Autodesk Inventor part; units mm, degrees
ref_plane "YZ Plane" through (0, 0, 0) normal (1, 0, 0) x (0, 1, 0)
ref_plane "XZ Plane" through (0, 0, 0) normal (0, 1, 0) x (-1, 0, 0)
ref_plane "XY Plane" through (0, 0, 0) normal (0, 0, 1) x (1, 0, 0)
sketch "Эскиз1" plane through (0, 0, 0) normal (1, 0, 0) x (0, 1, 0)
  line L0 (97.2644, 106.089) -> (-2.7356, 106.089)
  line L1 (-2.7356, 106.089) -> (-2.7356, -97.911)
  line L2 (-2.7356, -97.911) -> (97.2644, -97.911)
  line L3 (97.2644, -97.911) -> (97.2644, 106.089)
  line L4 (-2.7356, 106.089) -> (3.2644, 106.089)
  line L5 (3.2644, 106.089) -> (3.2644, 66.089)
  line L6 (3.2644, 66.089) -> (-2.7356, 66.089)
  line L7 (-2.7356, 66.089) -> (-2.7356, 106.089)
  line L8 (3.2644, 66.089) -> (-2.7356, 66.089)
  line L9 (-2.7356, 66.089) -> (-2.7356, 36.089)
  line L10 (-2.7356, 36.089) -> (3.2644, 36.089)
  line L11 (3.2644, 36.089) -> (3.2644, 66.089)
  line L12 (-2.7356, 36.089) -> (3.2644, 36.089)
  line L13 (3.2644, 36.089) -> (3.2644, -27.911)
  line L14 (3.2644, -27.911) -> (-2.7356, -27.911)
  line L15 (-2.7356, -27.911) -> (-2.7356, 36.089)
  line L16 (3.2644, -27.911) -> (-2.7356, -27.911)
  line L17 (-2.7356, -27.911) -> (-2.7356, -57.911)
  line L18 (-2.7356, -57.911) -> (3.2644, -57.911)
  line L19 (3.2644, -57.911) -> (3.2644, -27.911)
  line L20 (3.2644, -57.911) -> (-2.7356, -57.911)
  line L21 (-2.7356, -57.911) -> (-2.7356, -97.911)
  line L22 (-2.7356, -97.911) -> (3.2644, -97.911)
  line L23 (3.2644, -97.911) -> (3.2644, -57.911)
  line L24 (3.2644, 91.089) -> (-2.7356, 91.089)
  line L25 (-2.7356, 91.089) -> (-2.7356, 81.089)
  line L26 (-2.7356, 81.089) -> (3.2644, 81.089)
  line L27 (3.2644, 81.089) -> (3.2644, 91.089)
  line L28 (3.2644, -72.911) -> (-2.7356, -72.911)
  line L29 (-2.7356, -72.911) -> (-2.7356, -82.911)
  line L30 (-2.7356, -82.911) -> (3.2644, -82.911)
  line L31 (3.2644, -82.911) -> (3.2644, -72.911)
  point P0 (0, 0)
  point P1 (-2.7356, 66.089)
  point P2 (3.2644, 36.089)
  point P3 (-2.7356, -27.911)
  point P4 (0.2644, 91.089)
  point P5 (0.2644, 81.089)
  point P6 (0.2644, 66.089)
  point P7 (0.2644, -57.911)
  point P8 (0.2644, -72.911)
  point P9 (0.2644, -82.911)
  dimension "d0" = 204
  dimension "d1" = 100
  dimension "d2" = 40
  dimension "d3" = 30
  dimension "d4" = 30
  dimension "d5" = 40
  dimension "d8" = 6
  dimension "d41" = 10
  dimension "d42" = 15
  dimension "d43" = 15
  dimension "d44" = 10
extrude "Выдавливание1" add sketch "Эскиз1" along normal blind 6 contours L3 L2 L23 L19 L13 L11 L5 L0 | L5 L26 L1 L24 | L30 L1 L28 L23 | L11 L10 L1 L6 | L18 L1 L14 L19
sketch "Эскиз2" plane through (6, 0, 0) normal (1, 0, 0) x (0, 0, -1)
  line L0 (-106.089, 97.2644) -> (-106.089, 3.2644)
  line L1 (-106.089, 3.2644) -> (-100.089, 3.2644)
  line L2 (-100.089, 3.2644) -> (-100.089, 13.2644)
  line L3 (-100.089, 13.2644) -> (-106.089, 13.2644)
  line L4 (-106.089, 13.2644) -> (-106.089, 3.2644)
  line L5 (-106.089, 33.2644) -> (-100.089, 33.2644)
  line L6 (-100.089, 33.2644) -> (-100.089, 13.2644)
  line L7 (-100.089, 13.2644) -> (-106.089, 13.2644)
  line L8 (-106.089, 13.2644) -> (-106.089, 33.2644)
  line L9 (-100.089, 33.2644) -> (-106.089, 33.2644)
  line L10 (-106.089, 33.2644) -> (-106.089, 67.2644)
  line L11 (-106.089, 67.2644) -> (-100.089, 67.2644)
  line L12 (-100.089, 67.2644) -> (-100.089, 33.2644)
  line L13 (-100.089, 67.2644) -> (-106.089, 67.2644)
  line L14 (-106.089, 67.2644) -> (-106.089, 87.2644)
  line L15 (-106.089, 87.2644) -> (-100.089, 87.2644)
  line L16 (-100.089, 87.2644) -> (-100.089, 67.2644)
  line L17 (-100.089, 87.2644) -> (-106.089, 87.2644)
  line L18 (-106.089, 87.2644) -> (-106.089, 97.2644)
  line L19 (-106.089, 97.2644) -> (-100.089, 97.2644)
  line L20 (-100.089, 97.2644) -> (-100.089, 87.2644)
  line L21 (57.911, 3.2644) -> (97.911, 3.2644)
  line L22 (97.911, 3.2644) -> (91.911, 3.2644)
  line L23 (91.911, 3.2644) -> (91.911, 13.2644)
  line L24 (91.911, 13.2644) -> (97.911, 13.2644)
  line L25 (97.911, 13.2644) -> (97.911, 3.2644)
  line L26 (97.911, 13.2644) -> (91.911, 13.2644)
  line L27 (91.911, 13.2644) -> (91.911, 33.2644)
  line L28 (91.911, 33.2644) -> (97.911, 33.2644)
  line L29 (97.911, 33.2644) -> (97.911, 13.2644)
  line L30 (97.911, 33.2644) -> (91.911, 33.2644)
  line L31 (91.911, 33.2644) -> (91.911, 67.2644)
  line L32 (91.911, 67.2644) -> (97.911, 67.2644)
  line L33 (97.911, 67.2644) -> (97.911, 33.2644)
  line L34 (97.911, 67.2644) -> (91.911, 67.2644)
  line L35 (91.911, 67.2644) -> (91.911, 87.2644)
  line L36 (91.911, 87.2644) -> (97.911, 87.2644)
  line L37 (97.911, 87.2644) -> (97.911, 67.2644)
  line L38 (97.911, 87.2644) -> (91.911, 87.2644)
  line L39 (91.911, 87.2644) -> (91.911, 97.2644)
  line L40 (91.911, 97.2644) -> (97.911, 97.2644)
  line L41 (97.911, 97.2644) -> (97.911, 87.2644)
  point P0 (0, 0)
  point P1 (91.911, 3.2644)
  dimension "d9" = 10
  dimension "d10" = 20
  dimension "d11" = 10
  dimension "d12" = 20
  dimension "d13" = 34
  dimension "d14" = 6
  dimension "d15" = 10
  dimension "d16" = 20
  dimension "d17" = 20
  dimension "d18" = 10
  dimension "d19" = 34
  dimension "d20" = 6
extrude "Выдавливание2" cut sketch "Эскиз2" against normal through all contours L19 L20 L15 L0 | L11 L12 L5 L0 | L3 L2 L1 L0 | L23 L24 L25 L21 | L31 L32 L33 L28 | L39 L40 L41 L36
sketch "Эскиз4" plane through (6, 0, 0) normal (1, 0, 0) x (0, 0, -1)
  line L0 (-36.089, 3.2644) -> (27.911, 3.2644)
  line L1 (-19, 3.2644) -> (-16, 3.2644)
  line L2 (-16, 3.2644) -> (-16, 13.2644)
  line L3 (-16, 13.2644) -> (-19, 13.2644)
  line L4 (-19, 13.2644) -> (-19, 3.2644)
  line L5 (-21, 7.6644) -> (-14, 7.6644)
  line L6 (-14, 7.6644) -> (-14, 5.2644)
  line L7 (-14, 5.2644) -> (-21, 5.2644)
  line L8 (-21, 5.2644) -> (-21, 7.6644)
  line L9 (7, 3.2644) -> (4, 3.2644)
  line L10 (4, 3.2644) -> (4, 13.2644)
  line L11 (4, 13.2644) -> (7, 13.2644)
  line L12 (7, 13.2644) -> (7, 3.2644)
  line L13 (2, 7.6644) -> (9, 7.6644)
  line L14 (9, 7.6644) -> (9, 5.2644)
  line L15 (9, 5.2644) -> (2, 5.2644)
  line L16 (2, 5.2644) -> (2, 7.6644)
  point P0 (0, 0)
  point P1 (4, 5.2644)
  point P2 (4, 3.2644)
  point P3 (7, 5.2644)
  point P4 (7, 7.6644)
  point P5 (4, 7.6644)
  point P6 (-19, 5.2644)
  point P7 (-16, 3.2644)
  point P8 (-16, 5.2644)
  point P9 (-16, 7.6644)
  point P10 (-19, 7.6644)
  dimension "d26" = 7
  dimension "d27" = 7
  dimension "d28" = 2
  dimension "d29" = 3
  dimension "d30" = 2.4
  dimension "d31" = 10
  dimension "d32" = 16
  dimension "d33" = 2
  dimension "d34" = 2.4
  dimension "d35" = 2
  dimension "d36" = 3
  dimension "d37" = 10
  dimension "d38" = 4
extrude "Выдавливание4" cut sketch "Эскиз4" against normal blind 6.25
sketch "Эскиз6" plane through (6, 0, 0) normal (1, 0, 0) x (0, 0, -1)
  line L0 (91.911, 97.2644) -> (-100.089, 97.2644)
  line L1 (-4.089, 97.2644) -> (-4.089, 61.7663)
  line L2 (-100.089, 67.2644) -> (-100.089, 33.2644)
  line L3 (-100.089, 50.7644) -> (-90.089, 50.7644)
  line L4 (-90.089, 50.7644) -> (-90.089, 47.7644)
  line L5 (-90.089, 47.7644) -> (-100.089, 47.7644)
  line L6 (-100.089, 47.7644) -> (-100.089, 50.7644)
  line L7 (-98.089, 52.7644) -> (-95.689, 52.7644)
  line L8 (-95.689, 52.7644) -> (-95.689, 45.7644)
  line L9 (-95.689, 45.7644) -> (-98.089, 45.7644)
  line L10 (-98.089, 45.7644) -> (-98.089, 52.7644)
  line L11 (-91.089, -2.7356) -> (-81.089, -2.7356)
  line L12 (91.911, 50.7644) -> (81.911, 50.7644)
  line L13 (81.911, 50.7644) -> (81.911, 47.7644)
  line L14 (81.911, 47.7644) -> (91.911, 47.7644)
  line L15 (91.911, 47.7644) -> (91.911, 50.7644)
  line L16 (89.911, 52.7644) -> (87.511, 52.7644)
  line L17 (87.511, 52.7644) -> (87.511, 45.7644)
  line L18 (87.511, 45.7644) -> (89.911, 45.7644)
  line L19 (89.911, 45.7644) -> (89.911, 52.7644)
  point P0 (0, 0)
  point P1 (-96.889, 45.7644)
  point P2 (88.711, 45.7644)
  point P3 (89.911, 47.7644)
  point P4 (89.911, 50.7644)
  point P5 (87.511, 50.7644)
  point P6 (87.511, 47.7644)
  point P7 (-98.089, 50.7644)
  point P8 (-98.089, 47.7644)
  point P9 (-95.689, 47.7644)
  point P10 (-95.689, 50.7644)
  dimension "d45" = 7
  dimension "d46" = 3
  dimension "d47" = 2.4
  dimension "d48" = 2
  dimension "d49" = 2
  dimension "d50" = 10
  dimension "d51" = 50.5
extrude "Выдавливание5" cut sketch "Эскиз6" against normal blind 6
properties part number "перед"
The listing builds one solid part. Answer for the finished solid, in the listing's coordinates (mm). A direction names the side the tool comes from. Coordinates: 2 decimals unless noted, no trailing zeros. Order: outer loops, then holes, each group sorted by start corner. A loop starts at its lowest first (then second) coordinate and runs counter-clockwise, first axis right, second up.
Q1. Consider line 1 (Z direction, x = 4.25, y = 2); line 2 (Z direction, x = 4.15, y = 7); line 3 (Z direction, x = 2.8, y = 8.5). Determine where each line is inside the solid, lowest interval first.
Q2. For a pull along Z with two mould halves and no side action, classify faces 1 (the face through (3, 0, 66.089)), 2 (the face through (3, 8, -91.911)), 3 (the face through (6, 47, 6)) as pulls with the +Z half, pulls with the -Z half, needs draft (parallel to the pull), parting line crosses it, or undercut.
Q3. A cutting plane is placed at B-B, the plane y = 39. Write down the section's boundary in (x, z), and give its area (3 significant figures).
Q4. Which of the six approach directions +Z, -Z, +X, -X, +Y, -Y give full straight-line access (tool end or side, diameter ignored) to faces 4 (the face through (3, 59, 100.089)), 5 (the face through (3, 59, -91.911)), 6 (the face through (3, 92, -91.911)), 7 (the face through (3, 11, 19)), 8 (the face through (3, 3.264, 96))?
Q5. A cutting plane is placed at A-A, the plane z = 31.5. Write down the section's boundary in (x, y), and give its area (3 significant figures).
Q6. Given P1, Ø2, axis at x = 2.5, y = 4, coming from the -Z side; P2, Ø1.8, axis at x = 2.5, y = 92.5, coming from the +Z side; P3, Ø1.8, axis at x = 3.5, y = -0.5, coming from the +Z side, each flat-ended and moving along its own axis, determine where each tip first touches the part or whether it passes through.
Answers follow:
1. line 1: z = -82.91 to -72.91, -57.91 to -27.91, 36.09 to 66.09, 81.09 to 91.09
1. line 2: z = -91.91 to -9, -2 to 14, 21 to 100.09
1. line 3: z = -91.91 to -7, -4 to 16, 19 to 100.09
2. face 1: undercut
2. face 2: pulls with the -Z half
2. face 3: needs draft
3. outline: (0, -91.91) - (6, -91.91) - (6, 100.09) - (0, 100.09) - close
3. area: 1,150 mm2
4. face 4: +Z, +X, -X
4. face 5: -Z, +X, -X
4. face 6: -Z, +X, -X, +Y
4. face 7: +X, -X, -Y
4. face 8: +Z, +X, -X, -Y
5. outline: (0, 3.26) - (6, 3.26) - (6, 97.26) - (0, 97.26) - close
5. area: 564 mm2
6. P1: stops at z = -91.91
6. P2: stops at z = 100.09
6. P3: stops at z = 91.09
